Build history of the part. All positions in model axes, mm. Face numbers are marked on the shaded views. Round coordinates to 2 decimals unless told otherwise and drop trailing zeros. Order: outer loops, then holes, each group sorted by start corner. A loop starts at its lowest first (then second) coordinate and runs counter-clockwise, first axis right, second up. Notation, with made-up numbers: (17, 77) -> (74, 77) arc R25 cw to (74, 111) -> close; hole circle Ø4 at (27.25, -8). An arc over 180 degrees is marked (long way). Write item = value, one per line.
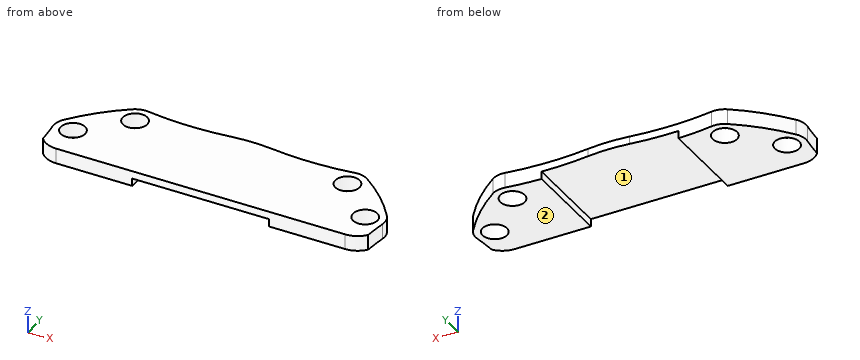
from build123d import *

# Parameters (mm, degrees)
SKETCH_1_R          = 1.6
EXTRUDE_1_DEPTH     = 2
SKETCH_2_W          = 18
SKETCH_2_H          = 1
CUT_EXTRUDE_1_DEPTH = 27.153393661
CUT_EXTRUDE_2_DEPTH = 33.316370891


with BuildPart() as part:
    # 草图1 → 凸台-拉伸1 (new body)
    with BuildSketch(Plane.XY):
        with BuildLine():
            Line((-19, 23.587026679), (19, 23.587026679))
            ThreePointArc((19, 23.587026679), (21.121320344, 22.708347023), (22, 20.587026679))
            Line((22, 20.587026679), (22, 12.587026679))
            ThreePointArc((22, 12.587026679), (21.121320344, 10.465706336), (19, 9.587026679))
            Line((19, 9.587026679), (-19, 9.587026679))
            ThreePointArc((-19, 9.587026679), (-21.121320344, 10.465706336), (-22, 12.587026679))
            Line((-22, 12.587026679), (-22, 20.587026679))
            ThreePointArc((-22, 20.587026679), (-21.121320344, 22.708347023), (-19, 23.587026679))
        make_face()
        with Locations((19.214153616, 13.959899742)):
            Circle(SKETCH_1_R, mode=Mode.SUBTRACT)
        with Locations((13.959899742, 19.214153616)):
            Circle(SKETCH_1_R, mode=Mode.SUBTRACT)
        with Locations((-13.959899742, 19.214153616)):
            Circle(SKETCH_1_R, mode=Mode.SUBTRACT)
        with Locations((-19.214153616, 13.959899742)):
            Circle(SKETCH_1_R, mode=Mode.SUBTRACT)
    extrude(amount=EXTRUDE_1_DEPTH)

    # 草图2 → 切除-拉伸1 (cut, through all)
    with BuildSketch(Plane.XZ.offset(-9.587026679)):
        with Locations((0, 0.5)):
            Rectangle(SKETCH_2_W, SKETCH_2_H)
    extrude(amount=-CUT_EXTRUDE_1_DEPTH, mode=Mode.SUBTRACT)

    # 草图3 → 切除-拉伸2 (cut, through all)
    with BuildSketch(Plane.XY.offset(2)):
        with BuildLine():
            Line((22, 12.587026679), (22, 20.587026679))
            ThreePointArc((22, 20.587026679), (21.121320344, 22.708347023), (19, 23.587026679))
            Line((19, 23.587026679), (-19, 23.587026679))
            ThreePointArc((-19, 23.587026679), (-21.121320344, 22.708347023), (-22, 20.587026679))
            Line((-22, 20.587026679), (-22, 12.587026679))
            ThreePointArc((-22, 12.587026679), (-21.838569798, 11.616191212), (-21.371652331, 10.749837189))
            ThreePointArc((-21.371652331, 10.749837189), (-21.504078669, 12.175448442), (-21.687439927, 13.595407183))
            ThreePointArc((-21.687439927, 13.595407183), (-21.641903091, 14.556584324), (-21.236696102, 15.429362873))
            ThreePointArc((-21.236696102, 15.429362873), (-18.561553006, 18.561553006), (-15.429362873, 21.236696102))
            ThreePointArc((-15.429362873, 21.236696102), (-14.556584324, 21.641903091), (-13.595407183, 21.687439927))
            ThreePointArc((-13.595407183, 21.687439927), (-8.168716079, 21.262073185), (-2.734521388, 21.577416267))
            ThreePointArc((-2.734521388, 21.577416267), (0, 21.75), (2.734521388, 21.577416267))
            ThreePointArc((2.734521388, 21.577416267), (8.168716079, 21.262073185), (13.595407183, 21.687439927))
            ThreePointArc((13.595407183, 21.687439927), (14.556584324, 21.641903091), (15.429362873, 21.236696102))
            ThreePointArc((15.429362873, 21.236696102), (18.561553006, 18.561553006), (21.236696102, 15.429362873))
            ThreePointArc((21.236696102, 15.429362873), (21.641903091, 14.556584324), (21.687439927, 13.595407183))
            ThreePointArc((21.687439927, 13.595407183), (21.504078669, 12.175448442), (21.371652331, 10.749837189))
            ThreePointArc((21.371652331, 10.749837189), (21.838569798, 11.616191212), (22, 12.587026679))
        make_face()
    extrude(amount=-CUT_EXTRUDE_2_DEPTH, mode=Mode.SUBTRACT)


solid = part.part
Q1. Mould opens along X. For the marked faces 1 and 2 say: released by +X, released by -X, zero draft, split by the parting line, or undercut.
Check values:
face_1 = undercut
face_2 = zero draft
Q2. Flat gauge pins, fed straight in: pin 1 (1.1 mm diameter, centred on y = 14.5, z = 0.5, fed in from -X); pin 2 (1.5 mm diameter, centred on x = 3, y = 12.5, fed in from -Z); pin 3 (0.5 mm diameter, centred on y = 15, z = 0.5, fed in from +X). Where does each tip first touch, or does it go through?
Check values:
pin_1 = -21.71
pin_2 = 1
pin_3 = 21.59
Q3. Probe probe 1 along X at (y, z) = (13.75, 1.35); probe 2 along X at (y, z) = (12.5, 0.6); probe 3 along X at (y, z) = (20.5, 1.55). List the from-to ranges inside material, lowest first.
Check values:
probe_1 = -21.71 to -20.8, -17.63 to 17.63, 20.8 to 21.71
probe_2 = -21.54 to -19.87, -18.56 to -9, 9 to 18.56, 19.87 to 21.54
probe_3 = -16.4 to -14.91, -13.01 to 13.01, 14.91 to 16.4
Q4. Cut at A-A, the plane x = -18. List the corners of the cut face in (y, z), and give its area (3 significant figures).
Check values:
outline = (9.59, 0) -> (12.92, 0) -> (12.92, 2) -> (9.59, 2) -> close; (15, 0) -> (19.11, 0) -> (19.11, 2) -> (15, 2) -> close
area = 14.9 mm²
Q5. Cut at C-C, the plane y = 18. List the corners of the cut face in (x, z), and give its area (3 significant figures).
Check values:
outline = (-19.11, 0) -> (-15, 0) -> (-15, 2) -> (-19.11, 2) -> close; (-12.92, 0) -> (-9, 0) -> (-9, 1) -> (9, 1) -> (9, 0) -> (12.92, 0) -> (12.92, 2) -> (-12.92, 2) -> close; (15, 0) -> (19.11, 0) -> (19.11, 2) -> (15, 2) -> close
area = 50.1 mm²
Q6. Cut at B-B, the plane z = 0.55. List the corners of the cut face in (x, y).
Check values:
outline = (-21.69, 13.6) arc R40 cw to (-21.37, 10.75) arc R3 ccw to (-19, 9.59) -> (-9, 9.59) -> (-9, 21.28) arc R40 cw to (-13.6, 21.69) arc R2.5 ccw to (-15.43, 21.24) arc R26.25 ccw to (-21.24, 15.43) arc R2.5 ccw to start; (9, 9.59) -> (19, 9.59) arc R3 ccw to (21.37, 10.75) arc R40 cw to (21.69, 13.6) arc R2.5 ccw to (21.24, 15.43) arc R26.25 ccw to (15.43, 21.24) arc R2.5 ccw to (13.6, 21.69) arc R40 cw to (9, 21.28) -> close; hole circle Ø3.2 at (-19.21, 13.96); hole circle Ø3.2 at (-13.96, 19.21); hole circle Ø3.2 at (13.96, 19.21); hole circle Ø3.2 at (19.21, 13.96)
Q7. Cut at D-D, the plane y = 16. List the corners of the cut face in (x, z).
Check values:
outline = (-20.81, 0) -> (-9, 0) -> (-9, 1) -> (9, 1) -> (9, 0) -> (20.81, 0) -> (20.81, 2) -> (-20.81, 2) -> close
